Verification items for this drawing (mm, ordinates from the low corner). Give positions to 0.01 mm unless a question says otherwise; leave off trailing zeros. Loops run counter-clockwise (first coordinate to the right, second up) from the corner with the lowest first, then second, coordinate; pieces in that order, holes last. Notation, with made-up numbers: (12.25, -13) -> (55.25, -13) arc R15 ccw to (55.25, -2) -> close; hole circle Ø9 at (23, 8.25). An arc over 180 degrees is marked (long way). Answer as CSV lines item,"result". Start each with the question number.
(1) Section check B-B on z = 3.5. State how many separate pieces and enclosed holes the cut face has, plus the area to 3 significant figures.
(2) Material ranges on line 1 (Y direction, x = 139.7, z = 1.5); line 2 (X direction, y = 11.75, z = 4); line 3 (X direction, y = 8.5, z = 6.25) (1 decimal), recorded low to high. Write a range as from..to.
(3) Section check C-C on y = 3.5. Enter the section's corners in (x, z) (1 decimal).
(4) Gauge pin test, flat end, axial feed: pin 1 Ø5.5 at (x, y) = (139.7, 9.525) entering from -Z. Record the tip position at first contact, or that the pin passes through.
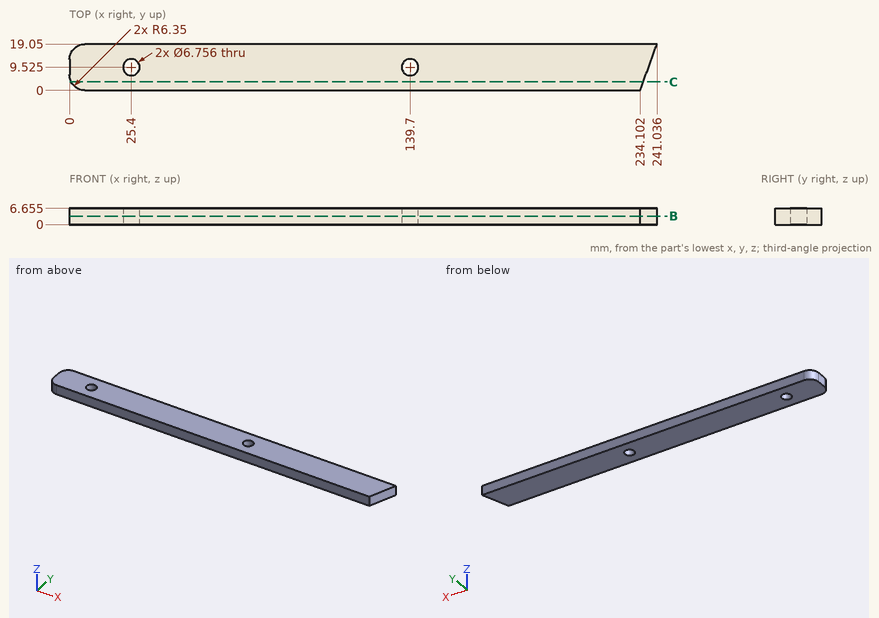
Working result:
1,separate pieces,"1"
1,enclosed holes,"2"
1,area,"4,440 mm^2"
2,line 1,"y = 0..6.15, 12.9..19.05"
2,line 2,"x = 0..22.86, 27.94..137.16, 142.24..238.38"
2,line 3,"x = 0..22.2, 28.6..136.5, 142.9..237.2"
3,outline,"(0.7, 0) -> (235.4, 0) -> (235.4, 6.7) -> (0.7, 6.7) -> close"
4,pin 1,"passes through"
